Autodesk Inventor part; units mm, degrees
ref_plane "YZ Plane" through (0, 0, 0) normal (1, 0, 0) x (0, 1, 0)
ref_plane "XZ Plane" through (0, 0, 0) normal (0, 1, 0) x (-1, 0, 0)
ref_plane "XY Plane" through (0, 0, 0) normal (0, 0, 1) x (1, 0, 0)
sketch "Sketch1" plane through (0, 0, 0) normal (0, 0, 1) x (1, 0, 0)
  circle A0 centre (0, 0) radius 6
  line L0 (10, 10) -> (10, -10)
  line L1 (10, -10) -> (-10, -10)
  line L2 (-10, -10) -> (-10, 10)
  line L3 (-10, 10) -> (10, 10)
  dimension "d0" = 12
  dimension "d1" = 20
extrude "Extrusion1" add sketch "Sketch1" along normal blind 20
sketch "Sketch2" plane through (-10, -10, 0) normal (0, -1, 0) x (1, 0, 0)
  line L0 (7.9561, 12.9375) -> (13.8857, 12.9375) construction
  line L1 (13.8857, 12.9375) -> (13.8857, 9.2988) construction
  line L2 (13.8857, 9.2988) -> (7.9561, 9.2988) construction
  line L3 (7.9561, 9.2988) -> (7.9561, 12.9375) construction
  point P0 (10, 0)
sketch "Sketch3" plane through (-10, -10, 0) normal (0, -1, 0) x (1, 0, 0)
  line L0 (0, 0) -> (0, 20)
  line L1 (20, 0) -> (20, 20)
  line L2 (0, 20) -> (-5, 20)
  line L3 (-5, 20) -> (-5, 0)
  line L4 (-5, 0) -> (0, 0)
  line L5 (0, 0) -> (0, 20)
  line L6 (20, 0) -> (20, 20)
  line L7 (20, 20) -> (25, 20)
  line L8 (25, 20) -> (25, 0)
  line L9 (25, 0) -> (20, 0)
  line L10 (20, 0) -> (20, 20)
  point P0 (10, 0)
  dimension "d4" = 30
extrude "Extrusion2" add sketch "Sketch3" against normal up to surface (20 mm away)
sketch "Sketch4" plane through (-15, -10, 0) normal (0, -1, 0) x (1, 0, 0)
  line L0 (21, 0) -> (21, 20)
  line L1 (9, 0) -> (9, 20)
  circle A0 centre (21, 10) radius 1.5
  point P0 (15, 0)
  dimension "d7" = 3
extrude "Extrusion3" cut sketch "Sketch4" against normal through all
properties part number "Bearing10" material "Acero, carbono"
The model under review builds one solid part; all positions refer to its coordinate system, in mm. Round coordinates to 2 decimals unless told otherwise and drop trailing zeros. Loops run counter-clockwise (first coordinate to the right, second up) from the corner with the lowest first, then second, coordinate; pieces in that order, holes last. Notation, with made-up numbers: M 6,19 L 43,19 A14 ccw 43,30 Z; hole C 48,-38 d10. An arc over 180 degrees is marked long. Put each result on its own line as item: value.
Q1. To check wall thickness, follow L1, parallel to Z at x = 6, y = -4; L2, parallel to Y at x = 0, z = 9; L3, parallel to X at y = -5.25, z = 10. State the ranges of each line that lie inside material, in increasing order.
Result set:
L1: z = 0 to 8.5, 11.5 to 20
L2: y = -10 to -6, 6 to 10
L3: x = -15 to -2.9, 2.9 to 4.5, 7.5 to 15
Q2. Consider section B-B, the plane x = 0. Give the boundary of the cut face in (y, z).
Result set:
outline: M -10,0 L -6,0 L -6,20 L -10,20 Z; M 6,0 L 10,0 L 10,20 L 6,20 Z
Q3. Consider section A-A, the plane y = 4. Give the boundary of the cut face in (x, z), then the cut area to 3 significant figures.
Result set:
outline: M -15,0 L -4.47,0 L -4.47,20 L -15,20 Z; M 4.47,0 L 15,0 L 15,20 L 4.47,20 Z; hole C 6,10 d3
area: 414 mm²
Q4. Mouldability with a two-part tool opening along Y and no side actions: class faces 1 (the flat face through (0, 10, 10)), 2 (the flat face through (-7, 0, 0)), 3 (the flat face through (0, -10, 10)), 4 (the cylindrical face through (-6, 0, 10)) as released by +Y, released by -Y, zero draft, split by the parting line, or undercut.
Result set:
face 1: released by +Y
face 2: zero draft
face 3: released by -Y
face 4: undercut
Q5. Consider section C-C, the plane z = 10. Give the boundary of the cut face in (x, y).
Result set:
outline: M -15,-10 L 4.5,-10 L 4.5,-3.97 A6 cw long 4.5,3.97 L 4.5,10 L -15,10 Z; M 7.5,-10 L 15,-10 L 15,10 L 7.5,10 Z
Q6. Consider section D-D, the plane y = 0. Give the boundary of the cut face in (x, z).
Result set:
outline: M -15,0 L -6,0 L -6,20 L -15,20 Z; M 6,0 L 15,0 L 15,20 L 6,20 L 6,11.5 A1.5 cw 6,8.5 Z
